Input: part model. Units: mm. Frame: model coordinates. A direction names the side the tool comes from. Coordinates: 2 decimals unless noted, no trailing zeros. Loops run counter-clockwise (first coordinate to the right, second up) from the corner with the lowest first, then second, coordinate; pieces in that order, holes last.
```python
from build123d import *

# Parameters (mm, degrees)
EXTRUDE_1_DEPTH     = 84
SKETCH_2_R          = 1.5
CUT_EXTRUDE_1_DEPTH = 87.948842416


with BuildPart() as part:
    # Эскиз1 → Бобышка-Вытянуть1 (new body)
    with BuildSketch(Plane.XY):
        with BuildLine():
            Line((-9.998476952, 0.174524064), (-19.998476952, 0.174524064))
            Line((-19.998476952, 0.174524064), (-19.998476952, 3.174524064))
            Line((-19.998476952, 3.174524064), (-12.998476952, 3.174524064))
            ThreePointArc((-12.998476952, 3.174524064), (0, 13.380508439), (12.998476952, 3.174524064))
            Line((12.998476952, 3.174524064), (19.998476952, 3.174524064))
            Line((19.998476952, 3.174524064), (19.998476952, 0.174524064))
            Line((19.998476952, 0.174524064), (9.998476952, 0.174524064))
            ThreePointArc((9.998476952, 0.174524064), (7.009092643, 7.132504492), (0, 10))
            ThreePointArc((0, 10), (-7.009092643, 7.132504492), (-9.998476952, 0.174524064))
        make_face()
    extrude(amount=EXTRUDE_1_DEPTH)

    # Эскиз2 → Вырез-Вытянуть1 (cut, through all)
    with BuildSketch(Plane(origin=(0, 3.174524064, 0), x_dir=(1, 0, 0), z_dir=(0, 1, 0))):
        with Locations(Location((-16.498476952, -21, 0), (0, 0, 270))):
            Circle(SKETCH_2_R)
        with Locations(Location((-16.498476952, -63, 0), (0, 0, 270))):
            Circle(SKETCH_2_R)
        with Locations(Location((16.498476952, -21, 0), (0, 0, 270))):
            Circle(SKETCH_2_R)
        with Locations(Location((16.498476952, -63, 0), (0, 0, 270))):
            Circle(SKETCH_2_R)
    extrude(amount=-CUT_EXTRUDE_1_DEPTH, mode=Mode.SUBTRACT)


solid = part.part
```
Item 1: Section query D-D (y = 4.75). Output: boundary loops of the cut face in (x, z).
Result:
outline: (-12.51, 0) - (-8.8, 0) - (-8.8, 84) - (-12.51, 84) - close; (8.8, 0) - (12.51, 0) - (12.51, 84) - (8.8, 84) - close
Item 2: Line query: L1, parallel to X at y = 1.35, z = 21; L2, parallel to X at y = 2.3, z = 21; L3, parallel to X at y = 6.75, z = 36. Output: solid intervals per line, ascending.
Result:
L1: x = -20 to -18, -15 to -9.91, 9.91 to 15, 18 to 20
L2: x = -20 to -18, -15 to -9.73, 9.73 to 15, 18 to 20
L3: x = -11.55 to -7.38, 7.38 to 11.55
Item 3: Reachability of faces 5 (the face through (16, 3.175, 41)), 6 (the face through (0, 11, 0)) from +Z, -Z, +X, -X, +Y, -Y: full face, straight path, thin tool, end or side. Return the list, or none.
Result:
face 5: +Z, -Z, +X, +Y
face 6: -Z, +X, -X, +Y, -Y
Item 4: Contact query for flat-ended pins moving along their axis: P1, Ø3.5, axis at x = -16.5, z = 21, coming from the +Y side; P2, Ø2.5, axis at x = 16.5, z = 21, coming from the +Y side; P3, Ø1.5, axis at y = 6, z = 42.5, coming from the -X side; P4, Ø8, axis at x = -10, z = 46.5, coming from the +Y side. Output: stop coordinate, or through.
Result:
P1: stops at y = 3.17
P2: passes through
P3: stops at x = -12.31
P4: stops at y = 11.96
Item 5: Section query B-B (y = 8.25). Output: boundary loops of the cut face in (x, z), then the cut area to 3 significant figures.
Result:
outline: (-10.53, 0) - (-5.65, 0) - (-5.65, 84) - (-10.53, 84) - close; (5.65, 0) - (10.53, 0) - (10.53, 84) - (5.65, 84) - close
area: 820 mm2
Item 6: Mould query, pull axis X, two halves, no side actions, for faces 1 (the face through (19.998, 2, 41)), 2 (the face through (16.95, 1.7, 64.43)), 3 (the face through (-16.05, 1.7, 64.43)), 4 (the face through (-17, 3.175, 41)). Classes: +X half, -X half, draft (parallel to the pull), parting line (faces both ways), or undercut.
Result:
face 1: +X half
face 2: undercut
face 3: undercut
face 4: draft
